from build123d import *

# Parameters (mm, degrees)
F0_R     = 1.2573
F1_DEPTH = 3


with BuildPart() as f1:
    # F0 (on Top) → F1 (new body)
    with BuildSketch(Plane.XY):
        Polygon((-4.835955, -42.675929), (-25.105155, -42.675929), (-25.105155, -60.836929), (-27.340355, -60.836929), (-27.340355, -72.622529), (-25.105155, -72.622529), (-25.105155, -97.819329), (-27.340355, -97.819329), (-27.340355, -109.604929), (-25.105155, -109.604929), (-25.105155, -128.350129), (31.790845, -128.350129), (31.790845, -109.604929), (34.026045, -109.604929), (34.026045, -97.819329), (31.790845, -97.819329), (31.790845, -72.622529), (34.026045, -72.622529), (34.026045, -60.836929), (31.790845, -60.836929), (31.790845, -42.675929), (9.489645, -42.675929), (9.489645, -57.687329), (-4.835955, -57.687329), align=None)
        with Locations((-22.107955, -103.839129)):
            Circle(F0_R, mode=Mode.SUBTRACT)
        with Locations((28.790845, -103.839129)):
            Circle(F0_R, mode=Mode.SUBTRACT)
        with Locations((-22.107955, -45.675929)):
            Circle(F0_R, mode=Mode.SUBTRACT)
        with Locations((28.790845, -45.675929)):
            Circle(F0_R, mode=Mode.SUBTRACT)
    extrude(amount=F1_DEPTH)


solid = f1.part
For this review, take the finished solid that the model builds, in its own axes (mm). A direction names the side the tool comes from. Give positions to 0.01 mm unless a question says otherwise; leave off trailing zeros. Loops run counter-clockwise (first coordinate to the right, second up) from the corner with the lowest first, then second, coordinate; pieces in that order, holes last. Notation, with made-up numbers: M 48.25,46 L 91.25,46 A19 ccw 91.25,81 Z; hole C -11,50.5 d1. An arc over 180 degrees is marked long. Put each result on its own line as item: value. Start each with the question number.
(1) Add section A-A, the plane y = -49. Write out the cut boundary in (x, z), then the cut area to 3 significant figures.
(2) For pin 1 (1.5 mm diameter, centred on y = -52.5, z = 2, fed in from +X); pin 2 (0.7 mm diameter, centred on x = -26, z = 2, fed in from +Y); pin 3 (0.9 mm diameter, centred on x = 4, z = 2, fed in from +Y), all flat-tipped, find the tip position at first contact; note any pin that passes through.
(3) Machinability: for faces 1 (the flat face through (33, -109.605, 1)), 2 (the flat face through (-25.105, -52, 1)), 3 (the flat face through (31.791, -85, 1)), which of the approach directions +Z, -Z, +X, -X, +Y, -Y give a long, thin tool a straight path to every point of the face, cutting with its end or side? Answer none if there is none.
(4) Wall thickness on L1, parallel to X at y = -104, z = 0.55; L2, parallel to X at y = -47.5, z = 0.3; L3, parallel to Y at x = -3.5, z = 2.5: over which ranges is each line inside the solid? List them lowest first.
(5) Add section B-B, the plane z = 1.7. Write out the cut boundary in (x, y), then the cut area to 3 significant figures.
(6) Add section C-C, the plane y = -90. Write out the cut boundary in (x, z).
Result:
1. outline: M -25.11,0 L -4.84,0 L -4.84,3 L -25.11,3 Z; M 9.49,0 L 31.79,0 L 31.79,3 L 9.49,3 Z
1. area: 128 mm^2
2. pin 1: stops at x = 31.79
2. pin 2: stops at y = -60.84
2. pin 3: stops at y = -57.69
3. face 1: +Z, -Z, +X, -Y
3. face 2: +Z, -Z, -X, +Y
3. face 3: +Z, -Z, +X
4. L1: x = -27.34 to -23.35, -20.86 to 27.54, 30.04 to 34.03
4. L2: x = -25.11 to -4.84, 9.49 to 31.79
4. L3: y = -128.35 to -57.69
5. outline: M -27.34,-109.6 L -25.11,-109.6 L -25.11,-128.35 L 31.79,-128.35 L 31.79,-109.6 L 34.03,-109.6 L 34.03,-97.82 L 31.79,-97.82 L 31.79,-72.62 L 34.03,-72.62 L 34.03,-60.84 L 31.79,-60.84 L 31.79,-42.68 L 9.49,-42.68 L 9.49,-57.69 L -4.84,-57.69 L -4.84,-42.68 L -25.11,-42.68 L -25.11,-60.84 L -27.34,-60.84 L -27.34,-72.62 L -25.11,-72.62 L -25.11,-97.82 L -27.34,-97.82 Z; hole C -22.11,-103.84 d2.51; hole C -22.11,-45.68 d2.51; hole C 28.79,-103.84 d2.51; hole C 28.79,-45.68 d2.51
5. area: 4,740 mm^2
6. outline: M -25.11,0 L 31.79,0 L 31.79,3 L -25.11,3 Z
